The drawing under review shows one solid part. Ordinate dimensions are in mm from its lowest x, y, z. Round coordinates to 2 decimals unless told otherwise and drop trailing zeros. Write each loop counter-clockwise with the first axis right and the second up, starting at its lowest first coordinate (ties: lowest second). Pieces come first, ordered by that corner, then holes.
Item 1: Add section A-A (x = 33.5). Give the boundary of the cut face in (y, z), plus the area to 3 significant figures.
Item 2: Add section D-D (y = 1.3). State how many separate pieces and enclosed holes the cut face has, plus the area to 3 significant figures.
Item 3: To check wall thickness, follow L1, parallel to X at y = 3.5, z = 55 (1 decimal); L2, parallel to X at y = 1, z = 315 (1 decimal); L3, parallel to Z at x = 83, y = 3.7. State the ranges of each line that lie inside material, in increasing order.
Item 4: Add section C-C (z = 188). Give the boundary of the cut face in (x, y) (1 decimal), plus the area to 3 significant figures.
Item 5: Clearance check with flat-ended pins moving along their axes: pin 1 Ø2 at (x, y) = (194, 4) entering from +Z; pin 2 Ø5 at (x, z) = (190.5, 81) entering from -Y; pin 3 Ø2.5 at (y, z) = (3, 284.5) entering from -X; pin 4 Ø2 at (x, y) = (46.5, 1.5) entering from -Z. State where each tip first meets the part, or that it passes through.
Item 6: Add section B-B (z = 34.5). Give the boundary of the cut face in (x, y) (1 decimal), plus the area to 3 significant figures.
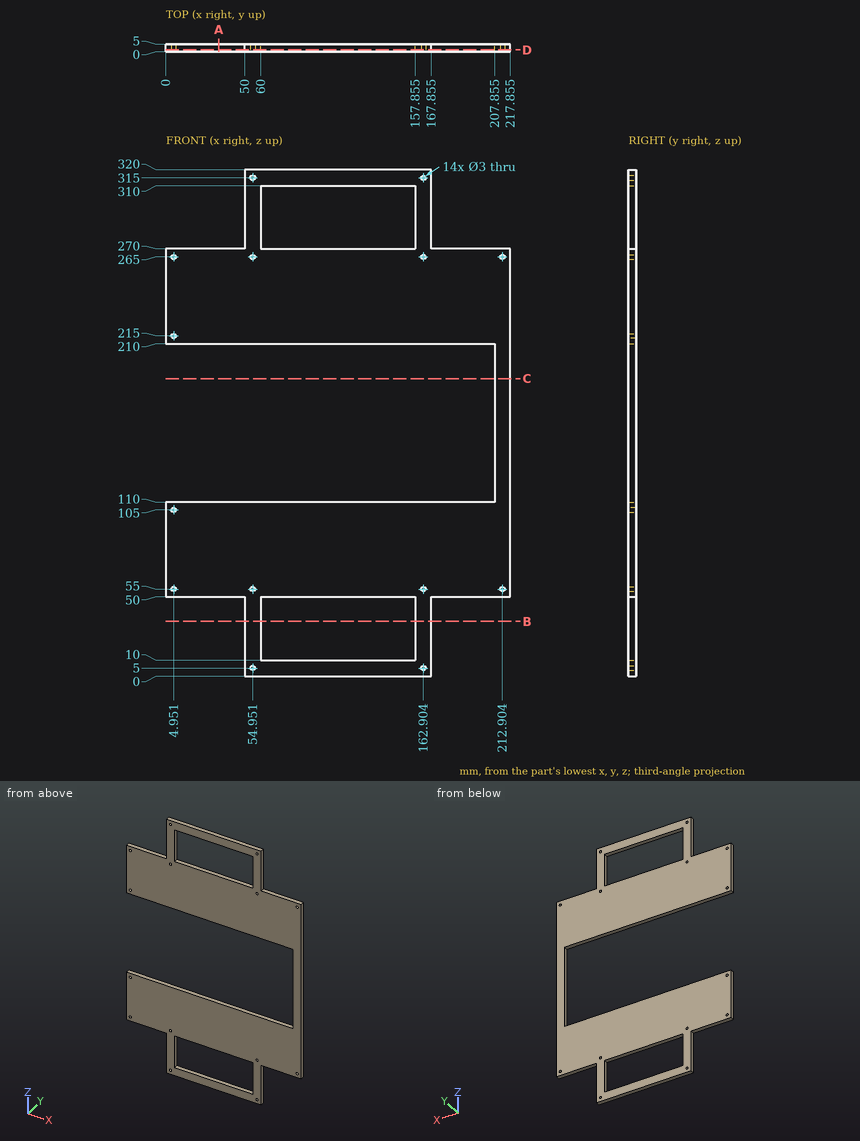
Numbers:
1. outline: (0, 50) - (5, 50) - (5, 110) - (0, 110) - close; (0, 210) - (5, 210) - (5, 270) - (0, 270) - close
1. area: 600 mm2
2. separate pieces: 1
2. enclosed holes: 16
2. area: 31,000 mm2
3. L1: x = 0 to 3.5, 6.5 to 53.5, 56.5 to 161.4, 164.4 to 211.4, 214.4 to 217.9
3. L2: x = 50 to 53.5, 56.5 to 161.4, 164.4 to 167.9
3. L3: z = 0 to 10, 50 to 110, 210 to 270, 310 to 320
4. outline: (207.9, 0) - (217.9, 0) - (217.9, 5) - (207.9, 5) - close
4. area: 50.0 mm2
5. pin 1: stops at z = 270
5. pin 2: stops at y = 0
5. pin 3: stops at x = 50
5. pin 4: stops at z = 50
6. outline: (50, 0) - (60, 0) - (60, 5) - (50, 5) - close; (157.9, 0) - (167.9, 0) - (167.9, 5) - (157.9, 5) - close
6. area: 100 mm2
